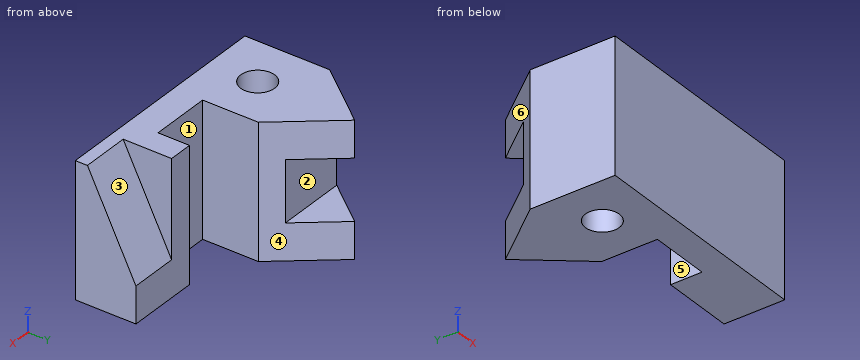
```python
from build123d import *

# Parameters (mm, degrees)
ESBO_O1_R                = 7
RESSALTO_EXTRUS_O1_DEPTH = 55
CORTE_EXTRUS_O1_REACH    = 127.707
ESBO_O2_W                = 25
ESBO_O2_H                = 18
CORTE_EXTRUS_O2_DEPTH    = 20


with BuildPart() as part:
    # Esboço1 → Ressalto-extrusão1 (new body)
    with BuildSketch(Plane.XY):
        Polygon((-86.062995877, 1.256505599), (-86.062995877, 36.256505599), (-66.062995877, 61.256505599), (-46.062995877, 36.256505599), (-46.062995877, 13.256505599), (-21.062995877, 13.256505599), (-21.062995877, 26.256505599), (8.937004123, 26.256505599), (8.937004123, 1.256505599), align=None)
        with Locations((-66.062995877, 21.256505599)):
            Circle(ESBO_O1_R, mode=Mode.SUBTRACT)
    extrude(amount=-RESSALTO_EXTRUS_O1_DEPTH)

    # Corte-extrusão1: up to this plane
    corte_extrus_o1_end = Plane(origin=(-66.062995877, 61.256505599, -55), z_dir=(0.7808688094430304, 0.6246950475544243, 0))
    # Esboço2 → Corte-extrusão1 (cut, up to the surface)
    with BuildSketch(Plane.ZY.offset(86.062995877), mode=Mode.PRIVATE) as corte_extrus_o1_sk1:
        with Locations((-27.5, 52.256505599)):
            Rectangle(ESBO_O2_W, ESBO_O2_H)
    corte_extrus_o1_tool1 = split(extrude(corte_extrus_o1_sk1.sketch, amount=-CORTE_EXTRUS_O1_REACH, mode=Mode.PRIVATE), bisect_by=corte_extrus_o1_end, keep=Keep.BOTH, mode=Mode.PRIVATE)
    add(corte_extrus_o1_tool1.solids().sort_by_distance((-86.062996, 52.256506, -27.5))[0], mode=Mode.SUBTRACT)

    # Esboço3 → Corte-extrusão2 (cut)
    with BuildSketch(Plane(origin=(8.937004123, 0, 0), x_dir=(0, 0, -1), z_dir=(1, 0, 0))):
        Polygon((0, 6.256505599), (40, 26.256505599), (0, 26.256505599), align=None)
    extrude(amount=-CORTE_EXTRUS_O2_DEPTH, mode=Mode.SUBTRACT)


solid = part.part
```
CAD build for the part. Positions are in the model's coordinates, mm. Face numbers are marked on the shaded views. A direction names the side the tool comes from. Round coordinates to 2 decimals unless told otherwise and drop trailing zeros. Write each loop counter-clockwise with the first axis right and the second up, starting at its lowest first coordinate (ties: lowest second). Pieces come first, ordered by that corner, then holes. Notation, with made-up numbers: M 86,-31 L 92,-31 A6 ccw 92,-27 Z; hole C 24,-15 d10. An arc over 180 degrees is marked long. One line per question, with ' | ' between items.
1. Cut at D-D on x = 1.5. Write the cut outline in (y, z), and give its area (3 significant figures).
Working result:
outline: M 1.26,-55 L 26.26,-55 L 26.26,-40 L 6.26,0 L 1.26,0 Z | area: 975 mm2
2. Mould opens along X. For the marked faces 4, 5 and 6 say: pulls with the +X half, pulls with the -X half, needs draft (parallel to the pull), parting line crosses it, or undercut.
Working result:
face 4: pulls with the +X half | face 5: undercut | face 6: pulls with the -X half
3. Cut at C-C on y = 55. Write the cut outline in (x, z), and give its area (3 significant figures).
Working result:
outline: M -71.07,-55 L -61.06,-55 L -61.06,-40 L -71.07,-40 Z; M -71.07,-15 L -61.06,-15 L -61.06,0 L -71.07,0 Z | area: 300 mm2
4. Cut at A-A on x = -72. Write the cut outline in (y, z), and give its area (3 significant figures).
Working result:
outline: M 1.26,-55 L 17.55,-55 L 17.55,0 L 1.26,0 Z; M 24.96,-55 L 53.84,-55 L 53.84,-40 L 43.26,-40 L 43.26,-15 L 53.84,-15 L 53.84,0 L 24.96,0 Z | area: 2,220 mm2
5. Which spindle directions (+Z, -Z, +X, -X, +Y, -Y) get a long thin tool onto all of the face, cutting with end or side? Do the marked faces 1, 2 and 3. Say none if no direction does.
Working result:
face 1: +Z, -Z, +Y | face 2: +X, -X, +Y | face 3: +Z, +X, +Y
6. Probe L1, parallel to Z at x = -61.5, y = 54.5; L2, parallel to X at y = 18.5, z = -17.5; L3, parallel to X at y = 15.5, z = -37. List the from-to ranges inside material, lowest first. Write a range as from..to.
Working result:
L1: -55..-40, -15..0 | L2: -86.06..-72.5, -59.63..-46.06, -21.06..-11.06 | L3: -86.06..-70.05, -62.08..-46.06, -21.06..8.94
7. Pin check, flat tips, straight feed: pin 1 Ø3 at (x, z) = (-73, -25.5) entering from +Y; pin 2 Ø20 at (x, z) = (-39.5, -18.5) entering from +Y; pin 3 Ø8.5 at (x, y) = (-66.06, 21.26) entering from +Z; pin 4 Ø5 at (x, z) = (-10, -11.5) entering from +Y. Stop position of each tip, or through.
Working result:
pin 1: y = 43.26 | pin 2: y = 40.55 | pin 3: through | pin 4: y = 26.26
8. Cut at B-B on z = -4.5. Write the cut outline in (x, y).
Working result:
outline: M -86.06,1.26 L 8.94,1.26 L 8.94,8.51 L -11.06,8.51 L -11.06,26.26 L -21.06,26.26 L -21.06,13.26 L -46.06,13.26 L -46.06,36.26 L -66.06,61.26 L -86.06,36.26 Z; hole C -66.06,21.26 d14
